from build123d import *

# Parameters (mm, degrees)
F4_W      = 63.5
F4_H      = 51
F4_R      = 1.5
F5_DEPTH  = 1.7
F6_W      = 51
F6_H      = 23
F7_DEPTH  = 17.3
F6_W_2    = 56
F6_H_2    = 6.75
F8_DEPTH  = 9
F6_W_3    = 4.45
F6_H_3    = 9
F9_DEPTH  = 5
F10_W     = 2
F10_H     = 2
F11_DEPTH = 4


with BuildPart() as f5:
    # F4 (on Top) → F5 (new body)
    with BuildSketch(Plane.XY):
        with Locations((22.1723487377, -2.2746226639)):
            Rectangle(F4_W, F4_H)
        with Locations((-7.0376512623, -12.0146226639)):
            Circle(F4_R, mode=Mode.SUBTRACT)
        with Locations((50.9623487377, -12.0146226639)):
            Circle(F4_R, mode=Mode.SUBTRACT)
        with Locations((-7.0376512623, 7.9853773361)):
            Circle(F4_R, mode=Mode.SUBTRACT)
        with Locations((50.9623487377, 7.9853773361)):
            Circle(F4_R, mode=Mode.SUBTRACT)
    extrude(amount=F5_DEPTH)

    # F6 (on face) → F7 (join)
    with BuildSketch(Plane.XY.offset(1.7)):
        with Locations((22.4463341404, -2.2746226639)):
            Rectangle(F6_W, F6_H)
    extrude(amount=F7_DEPTH)

    # F6 (on face) → F8 (join)
    with BuildSketch(Plane.XY.offset(1.7)):
        with Locations((22.4223487377, 15.8503773361)):
            Rectangle(F6_W_2, F6_H_2)
        with Locations((22.4223487377, -20.3996226639)):
            Rectangle(F6_W_2, F6_H_2)
    extrude(amount=F8_DEPTH)

    # F6 (on face) → F9 (join)
    with BuildSketch(Plane.XY.offset(1.7)):
        with Locations((-7.3526512623, -2.2746226639)):
            Rectangle(F6_W_3, F6_H_3)
    extrude(amount=F9_DEPTH)

    # F10 (on face) → F11 (join)
    with BuildSketch(Plane(origin=(-9.5776512623, 0, 0), x_dir=(0, -1, 0), z_dir=(-1, 0, 0))):
        with Locations((3.2746226639, 3.7837546077)):
            Rectangle(F10_W, F10_H)
    extrude(amount=F11_DEPTH)


solid = f5.part
Could you check a few things on this model? Use its own coordinates, in mm. A direction names the side the tool comes from. Coordinates: 2 decimals unless noted, no trailing zeros. Order: outer loops, then holes, each group sorted by start corner. A loop starts at its lowest first (then second) coordinate and runs counter-clockwise, first axis right, second up.
Q1. Suppose I cut it at B-B on y = -20.5. Please give me the cut outline in (x, z).
Q2. Suppose I cut it at D-D on y = 5.5. Please give me the cut outline in (x, z).
Q3. Please list where these lines run through material, in increasing order: L1, parallel to Y at x = 6, z = 8.25; L2, parallel to X at y = 1, z = 5.25; L3, parallel to X at y = -2.5, z = 3.25.
Q4. Will these pins go through, and if not, where does the flat tip stop? pin 1 (2 mm diameter, centred on x = -6.5, z = 3.5, fed in from +Y); pin 2 (1 mm diameter, centred on y = 16.5, z = 4.5, fed in from +X); pin 3 (0.6 mm diameter, centred on x = -11, y = -3.5, fed in from -Z); pin 4 (1 mm diameter, centred on x = 27.5, y = -6.5, fed in from -Z).
Q5. Suppose I cut it at A-A on z = 4. Please give me the cut outline in (x, y).
Q6. Which directions (+Z, -Z, +X, -X, +Y, -Y) give clear straight access to the entire face, cutting with the end or side of a thin tool? Please do faces 5 (the flat face through (-12, -2.275, 4)), 6 (the flat face through (22, -20, 10.7)), 7 (the flat face through (47.946, -2, 10)), 8 (the flat face through (22, -17.025, 6)).
Q7. Suppose I cut it at C-C on x = 5. Please give me the cut outline in (y, z).
Q8. Thinking about a two-plate mould opening in X: for faces 1 (the flat face through (-5.128, -2, 4)), 2 (the flat face through (22, 19.225, 6)), 3 (the cylindrical face through (-6.23, -10.75, 0.84)), 4 (the flat face through (-13.578, -3, 4)), which applies, released by +X, released by -X, zero draft, split by the parting line, or undercut?
Answer:
1. outline: (-9.58, 0) - (53.92, 0) - (53.92, 1.7) - (50.42, 1.7) - (50.42, 10.7) - (-5.58, 10.7) - (-5.58, 1.7) - (-9.58, 1.7) - close
2. outline: (-9.58, 0) - (53.92, 0) - (53.92, 1.7) - (47.95, 1.7) - (47.95, 19) - (-3.05, 19) - (-3.05, 1.7) - (-9.58, 1.7) - close
3. L1: y = -23.77 to -17.02, -13.77 to 9.23, 12.48 to 19.23
3. L2: x = -9.58 to -5.13, -3.05 to 47.95
3. L3: x = -13.58 to -5.13, -3.05 to 47.95
4. pin 1: stops at y = 19.23
4. pin 2: stops at x = 50.42
4. pin 3: stops at z = 2.78
4. pin 4: stops at z = 0
5. outline: (-13.58, -4.27) - (-9.58, -4.27) - (-9.58, -6.77) - (-5.13, -6.77) - (-5.13, 2.23) - (-9.58, 2.23) - (-9.58, -2.27) - (-13.58, -2.27) - close; (-5.58, -23.77) - (50.42, -23.77) - (50.42, -17.02) - (-5.58, -17.02) - close; (-5.58, 12.48) - (50.42, 12.48) - (50.42, 19.23) - (-5.58, 19.23) - close; (-3.05, -13.77) - (47.95, -13.77) - (47.95, 9.23) - (-3.05, 9.23) - close
6. face 5: +Z, -Z, -X, +Y
6. face 6: +Z, +X, -X, -Y
6. face 7: +Z, +X
6. face 8: +Z, +X, -X
7. outline: (-27.77, 0) - (23.23, 0) - (23.23, 1.7) - (19.23, 1.7) - (19.23, 10.7) - (12.48, 10.7) - (12.48, 1.7) - (9.23, 1.7) - (9.23, 19) - (-13.77, 19) - (-13.77, 1.7) - (-17.02, 1.7) - (-17.02, 10.7) - (-23.77, 10.7) - (-23.77, 1.7) - (-27.77, 1.7) - close
8. face 1: undercut
8. face 2: zero draft
8. face 3: undercut
8. face 4: released by -X
